Input: part model. Units: mm. Frame: model coordinates. A direction names the side the tool comes from. Coordinates: 2 decimals unless noted, no trailing zeros. Write each loop counter-clockwise with the first axis right and the second up, starting at its lowest first coordinate (ties: lowest second). Pieces come first, ordered by that corner, then holes. Notation, with made-up numbers: (72, 55) - (82, 55) arc R20 cw to (82, 67) - close; hole circle Ø6 at (68.5, 7.25). An arc over 180 degrees is marked (long way). One line per question, with ' | ' between items. Start each with the question number.
1) Section query C-C on x = 6.5. Return loops of the section in (y, z), and give its area (3 significant figures).
2) First-contact query: P1, Ø2, axis at x = 25.5, z = -23, coming from the +Y side; P2, Ø5, axis at x = 11, z = 3.5, coming from the -Y side; P3, Ø1, axis at x = 26, z = 22.5, coming from the -Y side. Flat tips, straight axial feed; report the tip coordinate or a pass-through.
3) Line query: line 1 (Y direction, x = 26.25, z = 23.5); line 2 (X direction, y = -20, z = 4.5); line 3 (Y direction, x = 17.5, z = -0.5). Output: solid intervals per line, ascending.
4) Section query D-D on z = 23. Return loops of the section in (x, y), and give its area (3 significant figures).
5) Reachability of faces 1 (the flat face through (25, -15, -10)), 2 (the flat face through (26, 10.105, -23)), 3 (the flat face through (26, -9.983, 23)), 4 (the flat face through (26, -9.983, -23)) from +Z, -Z, +X, -X, +Y, -Y: full face, straight path, thin tool, end or side. Return the list, or none.
6) Section query B-B on z = 0. Return loops of the section in (x, y).
7) Section query A-A on y = 0. Return loops of the section in (x, z).
```python
from build123d import *

# Parameters (mm, degrees)
SKETCH_2_R      = 17.5
EXTRUDE_1_DEPTH = 25
EXTRUDE_2_DEPTH = 2


with BuildPart() as part:
    # 草图2 → 凸台-拉伸1 (new body)
    with BuildSketch(Plane(origin=(0, 0, 0), x_dir=(0, 0, -1), z_dir=(1, 0, 0))):
        Circle(SKETCH_2_R)
    extrude(amount=EXTRUDE_1_DEPTH)

    # 草图3 → 凸台-拉伸2 (add)
    with BuildSketch(Plane(origin=(25, 0, 0), x_dir=(0, 0, -1), z_dir=(1, 0, 0))):
        with BuildLine():
            Line((-22.296317142, 10.105406997), (-19.874770628, 10.105406997))
            ThreePointArc((-19.874770628, 10.105406997), (0, 22.296317142), (19.874770628, 10.105406997))
            Line((19.874770628, 10.105406997), (22.296317142, 10.105406997))
            Line((22.296317142, 10.105406997), (26.334302173, 10.105406997))
            Line((26.334302173, 10.105406997), (26.334302173, 0))
            Line((26.334302173, 0), (26.334302173, -9.98295184))
            Line((26.334302173, -9.98295184), (22.296317142, -9.98295184))
            Line((22.296317142, -9.98295184), (19.936560151, -9.98295184))
            ThreePointArc((19.936560151, -9.98295184), (0, -22.296317142), (-19.936560151, -9.98295184))
            Line((-19.936560151, -9.98295184), (-22.296317142, -9.98295184))
            Line((-22.296317142, -9.98295184), (-26.374870703, -9.98295184))
            Line((-26.374870703, -9.98295184), (-26.374870703, 0))
            Line((-26.374870703, 0), (-26.374870703, 10.105406997))
            Line((-26.374870703, 10.105406997), (-22.296317142, 10.105406997))
        make_face()
    extrude(amount=EXTRUDE_2_DEPTH)


solid = part.part
```
Answer key:
1) outline: circle Ø35 at (0, 0) | area: 962 mm²
2) P1: y = 10.11 | P2: y = -17.47 | P3: y = -9.98
3) line 1: -9.98 to 10.11 | line 2: 25 to 27 | line 3: -17.49 to 17.49
4) outline: (25, -9.98) - (27, -9.98) - (27, 10.11) - (25, 10.11) - close | area: 40.2 mm²
5) face 1: -X | face 2: -Z, +X, -X, +Y | face 3: +Z, +X, -X, -Y | face 4: -Z, +X, -X, -Y
6) outline: (0, -17.5) - (25, -17.5) - (25, -22.3) - (27, -22.3) - (27, 22.3) - (25, 22.3) - (25, 17.5) - (0, 17.5) - close
7) outline: (0, -17.5) - (25, -17.5) - (25, -26.33) - (27, -26.33) - (27, 26.37) - (25, 26.37) - (25, 17.5) - (0, 17.5) - close
